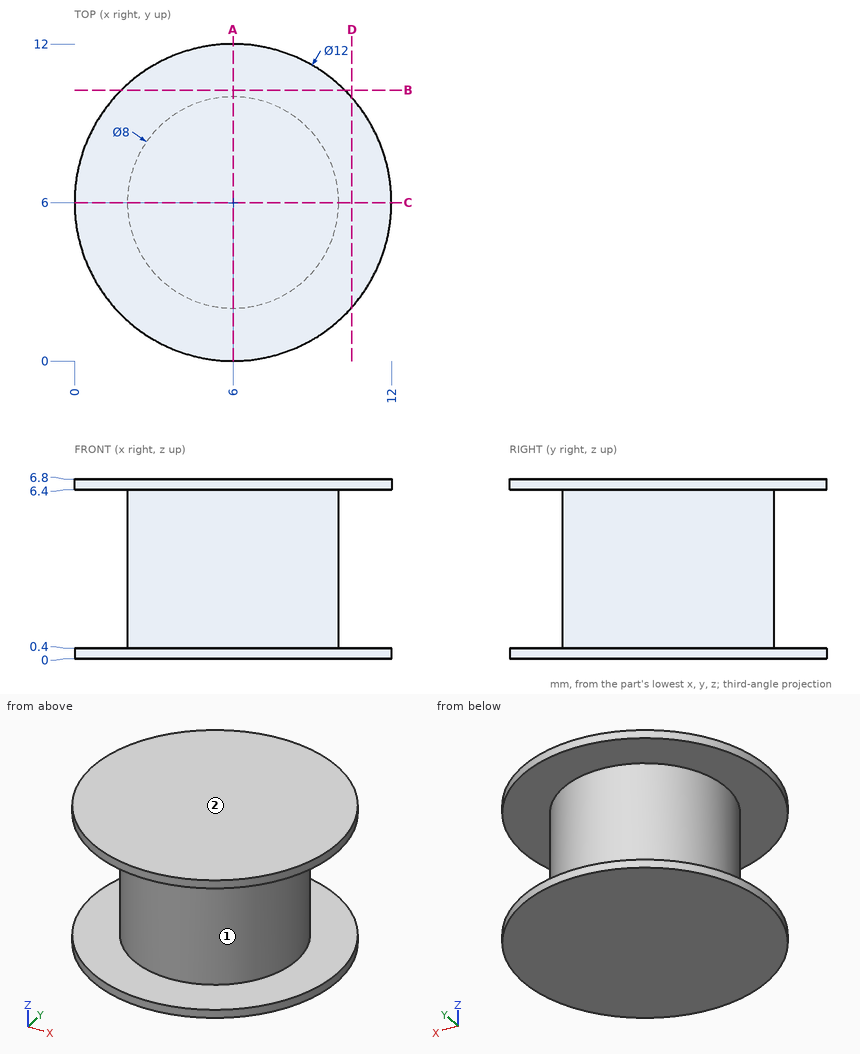
Verification items for this drawing (mm, ordinates from the low corner). A direction names the side the tool comes from. Coordinates: 2 decimals unless noted, no trailing zeros. Write each loop counter-clockwise with the first axis right and the second up, starting at its lowest first coordinate (ties: lowest second). Pieces come first, ordered by that corner, then holes. Notation, with made-up numbers: (14, -31) -> (23, -31) arc R16 cw to (23, -19) -> close; hole circle Ø5 at (0.25, 21.5). An arc over 180 degrees is marked (long way). One line per item, written item: value. Start each with the question number.
Q1. Go/stop test with flat-tipped pins: P1, Ø2, axis at x = 2, z = 2, coming from the +Y side; P2, Ø1, axis at y = 8, z = 4.5, coming from the -X side; P3, Ø4, axis at x = 8, z = 2, coming from the -Y side. Record where each tip stops, or that it passes through.
Q2. Thickness scan on L1, parallel to Z at x = 10.25, y = 2; L2, parallel to Y at x = 6, z = 3. Record the ranges inside material, lowest first. Write a range as from..to.
Q3. Access from +Z, -Z, +X, -X, +Y, -Y to the whole of each face (thin tool, end or side, straight path). Record for the marked faces 1 and 2.
Q4. Cross-section at A-A on x = 6. Enter the section's corners in (y, z), and give its area (3 significant figures).
Q5. Cross-section at D-D on x = 10.5. Enter the section's corners in (y, z), and give its area (3 significant figures).
Q6. Cross-section at B-B on y = 10.25. Enter the section's corners in (x, z), and give its area (3 significant figures).
Checked values:
1. P1: stops at y = 8.65
1. P2: stops at x = 2.29
1. P3: stops at y = 0.05
2. L1: z = 0..0.4, 6.4..6.8
2. L2: y = 2..10
3. face 1: none
3. face 2: +Z, +X, -X, +Y, -Y
4. outline: (0, 0) -> (12, 0) -> (12, 0.4) -> (10, 0.4) -> (10, 6.4) -> (12, 6.4) -> (12, 6.8) -> (0, 6.8) -> (0, 6.4) -> (2, 6.4) -> (2, 0.4) -> (0, 0.4) -> close
4. area: 57.6 mm²
5. outline: (2.03, 0) -> (9.97, 0) -> (9.97, 0.4) -> (2.03, 0.4) -> close; (2.03, 6.4) -> (9.97, 6.4) -> (9.97, 6.8) -> (2.03, 6.8) -> close
5. area: 6.35 mm²
6. outline: (1.76, 0) -> (10.24, 0) -> (10.24, 0.4) -> (1.76, 0.4) -> close; (1.76, 6.4) -> (10.24, 6.4) -> (10.24, 6.8) -> (1.76, 6.8) -> close
6. area: 6.78 mm²
